Could you check a few things on this model? Use its own coordinates, in mm. A direction names the side the tool comes from. Give positions to 0.01 mm unless a question says otherwise; leave off trailing zeros. Loops run counter-clockwise (first coordinate to the right, second up) from the corner with the lowest first, then second, coordinate; pieces in that order, holes last. Notation, with made-up numbers: (-8, -27.5) -> (16, -27.5) arc R26 cw to (16, -8.5) -> close; hole circle Ø4 at (6.25, 21). An arc over 180 degrees is marked (long way). Write item = value, one per line. Start each with the question number.
1) I want a section at A-A (z = 8). List the corners of the cut face in (x, y) for me, and give its area (3 significant figures).
2) If we mould it in two halves opening along Y, with no side actions, what happens to faces 1 (the face through (17.3, -31.38, -17.42)), 2 (the face through (3, -33, -22)), 3 (the face through (14.026, 33.377, 10.944))? For each: +Y half, -Y half, draft (parallel to the pull), parting line (faces both ways), or undercut.
3) On a 3-axis mill with a long thin cutter (end or side, diameter ignored), from which of +Z, -Z, +X, -X, +Y, -Y can I reach the whole of each face in a straight line? I mean faces 4 (the face through (-17, 27, 15)), 5 (the face through (17.3, -31.38, 17.58)), 6 (the face through (-31.64, -11.92, 10.94)). Say none if no direction works.
4) I'm going to push flat-ended pins straight in: pin 1 Ø12 at (y, z) = (3, -14.5) entering from +X; pin 2 Ø2 at (y, z) = (28, -16.5) entering from +X; pin 3 Ø1.5 at (x, y) = (29.5, 11.5) entering from -Z. Where does each tip first touch, or does it pass through?
5) I need wall thicknesses on probe 1 along Z at (x, y) = (-17.5, -36.5); probe 2 along X at (y, z) = (0, 11); probe 3 along Y at (x, z) = (15, 10.5). Which ranges of each line are inside material? Lowest first, please. Write a range as from..to.
from build123d import *

# Parameters (mm, degrees)
EXTRUSION1_DEPTH              = 15
EXTRUSION1_DEPTH_BACK         = 15
SKETCH1_R                     = 37.5
SKETCH1_R_2                   = 31.15
CIRPATTERN1_COUNT             = 27
HOLE4_D                       = 2.5
HOLE4_DEPTH                   = 8
HOLE4_TIP                     = 1.25
EXTRUSION11_START             = 7
SKETCH5_R                     = 37.5
SKETCH5_R_2                   = 32.5
EXTRUSION11_DEPTH             = 7
SKETCH6_R                     = 37.5
SKETCH6_R_2                   = 32.5
EXTRUSION17_DEPTH             = 7
EXTRUSION18_REACH             = 59.415
EXTRUSION18_DIRECTION_2_REACH = 59.415
FILLET5_R                     = 20
HOLE6_D                       = 2.5
HOLE6_DEPTH                   = 8
HOLE6_TIP                     = 0.751075774


with BuildPart() as part:
    # Sketch1 → Extrusion1 (new, two sides: drawn at the far end of the back side and taken through both)
    with BuildSketch(Plane.XY.offset(-EXTRUSION1_DEPTH_BACK)):
        Circle(SKETCH1_R)
        Circle(SKETCH1_R_2, mode=Mode.SUBTRACT)
    extrusion1 = extrude(amount=EXTRUSION1_DEPTH + EXTRUSION1_DEPTH_BACK)


with BuildPart() as cirpattern1_1:
    # CirPattern1: pattern copy
    add(extrusion1.rotate(Axis((0, 0, 80.9), (0, 0, -1)), 1 * 360 / CIRPATTERN1_COUNT))


with BuildPart() as cirpattern1_2:
    # CirPattern1: pattern copy
    add(extrusion1.rotate(Axis((0, 0, 80.9), (0, 0, -1)), 2 * 360 / CIRPATTERN1_COUNT))


with BuildPart() as cirpattern1_3:
    # CirPattern1: pattern copy
    add(extrusion1.rotate(Axis((0, 0, 80.9), (0, 0, -1)), 3 * 360 / CIRPATTERN1_COUNT))


with BuildPart() as cirpattern1_4:
    # CirPattern1: pattern copy
    add(extrusion1.rotate(Axis((0, 0, 80.9), (0, 0, -1)), 4 * 360 / CIRPATTERN1_COUNT))


with BuildPart() as cirpattern1_5:
    # CirPattern1: pattern copy
    add(extrusion1.rotate(Axis((0, 0, 80.9), (0, 0, -1)), 5 * 360 / CIRPATTERN1_COUNT))


with BuildPart() as cirpattern1_6:
    # CirPattern1: pattern copy
    add(extrusion1.rotate(Axis((0, 0, 80.9), (0, 0, -1)), 6 * 360 / CIRPATTERN1_COUNT))


with BuildPart() as cirpattern1_7:
    # CirPattern1: pattern copy
    add(extrusion1.rotate(Axis((0, 0, 80.9), (0, 0, -1)), 7 * 360 / CIRPATTERN1_COUNT))


with BuildPart() as cirpattern1_8:
    # CirPattern1: pattern copy
    add(extrusion1.rotate(Axis((0, 0, 80.9), (0, 0, -1)), 8 * 360 / CIRPATTERN1_COUNT))


with BuildPart() as cirpattern1_9:
    # CirPattern1: pattern copy
    add(extrusion1.rotate(Axis((0, 0, 80.9), (0, 0, -1)), 9 * 360 / CIRPATTERN1_COUNT))


with BuildPart() as cirpattern1_10:
    # CirPattern1: pattern copy
    add(extrusion1.rotate(Axis((0, 0, 80.9), (0, 0, -1)), 10 * 360 / CIRPATTERN1_COUNT))


with BuildPart() as cirpattern1_11:
    # CirPattern1: pattern copy
    add(extrusion1.rotate(Axis((0, 0, 80.9), (0, 0, -1)), 11 * 360 / CIRPATTERN1_COUNT))


with BuildPart() as cirpattern1_12:
    # CirPattern1: pattern copy
    add(extrusion1.rotate(Axis((0, 0, 80.9), (0, 0, -1)), 12 * 360 / CIRPATTERN1_COUNT))


with BuildPart() as cirpattern1_13:
    # CirPattern1: pattern copy
    add(extrusion1.rotate(Axis((0, 0, 80.9), (0, 0, -1)), 13 * 360 / CIRPATTERN1_COUNT))


with BuildPart() as cirpattern1_14:
    # CirPattern1: pattern copy
    add(extrusion1.rotate(Axis((0, 0, 80.9), (0, 0, -1)), 14 * 360 / CIRPATTERN1_COUNT))


with BuildPart() as cirpattern1_15:
    # CirPattern1: pattern copy
    add(extrusion1.rotate(Axis((0, 0, 80.9), (0, 0, -1)), 15 * 360 / CIRPATTERN1_COUNT))


with BuildPart() as cirpattern1_16:
    # CirPattern1: pattern copy
    add(extrusion1.rotate(Axis((0, 0, 80.9), (0, 0, -1)), 16 * 360 / CIRPATTERN1_COUNT))


with BuildPart() as cirpattern1_17:
    # CirPattern1: pattern copy
    add(extrusion1.rotate(Axis((0, 0, 80.9), (0, 0, -1)), 17 * 360 / CIRPATTERN1_COUNT))


with BuildPart() as cirpattern1_18:
    # CirPattern1: pattern copy
    add(extrusion1.rotate(Axis((0, 0, 80.9), (0, 0, -1)), 18 * 360 / CIRPATTERN1_COUNT))


with BuildPart() as cirpattern1_19:
    # CirPattern1: pattern copy
    add(extrusion1.rotate(Axis((0, 0, 80.9), (0, 0, -1)), 19 * 360 / CIRPATTERN1_COUNT))


with BuildPart() as cirpattern1_20:
    # CirPattern1: pattern copy
    add(extrusion1.rotate(Axis((0, 0, 80.9), (0, 0, -1)), 20 * 360 / CIRPATTERN1_COUNT))


with BuildPart() as cirpattern1_21:
    # CirPattern1: pattern copy
    add(extrusion1.rotate(Axis((0, 0, 80.9), (0, 0, -1)), 21 * 360 / CIRPATTERN1_COUNT))


with BuildPart() as cirpattern1_22:
    # CirPattern1: pattern copy
    add(extrusion1.rotate(Axis((0, 0, 80.9), (0, 0, -1)), 22 * 360 / CIRPATTERN1_COUNT))


with BuildPart() as cirpattern1_23:
    # CirPattern1: pattern copy
    add(extrusion1.rotate(Axis((0, 0, 80.9), (0, 0, -1)), 23 * 360 / CIRPATTERN1_COUNT))


with BuildPart() as cirpattern1_24:
    # CirPattern1: pattern copy
    add(extrusion1.rotate(Axis((0, 0, 80.9), (0, 0, -1)), 24 * 360 / CIRPATTERN1_COUNT))


with BuildPart() as cirpattern1_25:
    # CirPattern1: pattern copy
    add(extrusion1.rotate(Axis((0, 0, 80.9), (0, 0, -1)), 25 * 360 / CIRPATTERN1_COUNT))


with BuildPart() as cirpattern1_26:
    # CirPattern1: pattern copy
    add(extrusion1.rotate(Axis((0, 0, 80.9), (0, 0, -1)), 26 * 360 / CIRPATTERN1_COUNT))


with BuildPart() as part_1:
    add(part.part)

    # CirPattern1 united with what the copies: union CirPattern1_1, CirPattern1_2, CirPattern1_3, CirPattern1_4, CirPattern1_5, CirPattern1_6, CirPattern1_7, CirPattern1_8, CirPattern1_9, CirPattern1_10, CirPattern1_11, CirPattern1_12, CirPattern1_13, CirPattern1_14, CirPattern1_15, CirPattern1_16, CirPattern1_17, CirPattern1_18, CirPattern1_19, CirPattern1_20, CirPattern1_21, CirPattern1_22, CirPattern1_23, CirPattern1_24, CirPattern1_25, CirPattern1_26
    add(cirpattern1_1.part)
    add(cirpattern1_2.part)
    add(cirpattern1_3.part)
    add(cirpattern1_4.part)
    add(cirpattern1_5.part)
    add(cirpattern1_6.part)
    add(cirpattern1_7.part)
    add(cirpattern1_8.part)
    add(cirpattern1_9.part)
    add(cirpattern1_10.part)
    add(cirpattern1_11.part)
    add(cirpattern1_12.part)
    add(cirpattern1_13.part)
    add(cirpattern1_14.part)
    add(cirpattern1_15.part)
    add(cirpattern1_16.part)
    add(cirpattern1_17.part)
    add(cirpattern1_18.part)
    add(cirpattern1_19.part)
    add(cirpattern1_20.part)
    add(cirpattern1_21.part)
    add(cirpattern1_22.part)
    add(cirpattern1_23.part)
    add(cirpattern1_24.part)
    add(cirpattern1_25.part)
    add(cirpattern1_26.part)

    # Hole4
    with Locations(Plane.XY.offset(15)):
        with Locations((35, 0), (13.862791811, 32.137563741), (-24.018457325, 25.458077455), (-32.889241728, -11.970705016), (-2.035069012, -34.940785539), (31.277142411, -15.707971307)):
            Hole(HOLE4_D / 2, depth=HOLE4_DEPTH)
            with Locations((0, 0, -(HOLE4_DEPTH + HOLE4_TIP / 2))):  # 90° drill point
                Cone(0, HOLE4_D / 2, HOLE4_TIP, mode=Mode.SUBTRACT)

    # Sketch5 → Extrusion11 (add)
    with BuildSketch(Plane(origin=(0, 0, -15), x_dir=(-1, 0, 0), z_dir=(0, 0, -1)).offset(EXTRUSION11_START)):
        with Locations(Location((0, 0, 0), (0, 0, 180))):
            Circle(SKETCH5_R)
        Circle(SKETCH5_R_2, mode=Mode.SUBTRACT)
    extrude(amount=-EXTRUSION11_DEPTH)

    # Sketch6 → Extrusion17 (add)
    with BuildSketch(Plane.XY.offset(15)):
        Circle(SKETCH6_R)
        with Locations(Location((0, 0, 0), (0, 0, 180))):
            Circle(SKETCH6_R_2, mode=Mode.SUBTRACT)
    extrude(amount=EXTRUSION17_DEPTH)

    # Extrusion18: up to this face of the body (flat: up to its plane)
    extrusion18_end = Plane(part_1.part.faces().sort_by_distance((-36.439339828, 0, 22))[0])
    # Sketch7 → Extrusion18 (add, up to the picked face)
    with BuildSketch(Plane.XY, mode=Mode.PRIVATE) as extrusion18_sk1:
        with BuildLine():
            Line((22.5, -40), (-22.5, -40))
            Line((-22.5, -40), (-22.5, -30))
            ThreePointArc((-22.5, -30), (0, -37.5), (22.5, -30))
            Line((22.5, -30), (22.5, -40))
        make_face()
    extrusion18_tool1 = split(extrude(extrusion18_sk1.sketch, amount=EXTRUSION18_REACH, mode=Mode.PRIVATE), bisect_by=extrusion18_end, keep=Keep.BOTH, mode=Mode.PRIVATE)
    add(extrusion18_tool1.solids().sort_by(Axis((22.039023, -35, 0), (0, 0, 1)))[0])

    # Extrusion18 direction 2: up to this face of the body (flat: up to its plane)
    extrusion18_direction_2_end = Plane(part_1.part.faces().sort_by_distance((-36.439339828, 0, -22))[0])
    # Sketch7 → Extrusion18 direction 2 (add, up to the picked face)
    with BuildSketch(Plane.XY, mode=Mode.PRIVATE) as extrusion18_direction_2_sk1:
        with BuildLine():
            Line((22.5, -40), (-22.5, -40))
            Line((-22.5, -40), (-22.5, -30))
            ThreePointArc((-22.5, -30), (0, -37.5), (22.5, -30))
            Line((22.5, -30), (22.5, -40))
        make_face()
    extrusion18_direction_2_tool1 = split(extrude(extrusion18_direction_2_sk1.sketch, amount=-EXTRUSION18_DIRECTION_2_REACH, mode=Mode.PRIVATE), bisect_by=extrusion18_direction_2_end, keep=Keep.BOTH, mode=Mode.PRIVATE)
    add(extrusion18_direction_2_tool1.solids().sort_by(Axis((22.039023, -35, 0), (0, 0, -1)))[0])

    # Fillet5
    fillet5_edges = [part_1.edges().sort_by_distance(p)[0] for p in [
        (22.5, -30, 0),
        (-22.5, -30, 0),
    ]]
    fillet(fillet5_edges, radius=FILLET5_R)

    # Sketch8 → Revolution1 (revolve, cut)
    with BuildSketch(Plane.YZ, mode=Mode.PRIVATE) as revolution1_sk:
        Polygon((31.493036454, 15), (30.493036454, 15), (30.493036454, 14), align=None)
    revolution1 = revolve(revolution1_sk.sketch.rotate(Axis((0, 0, 0), (0, 0, 1)), 270), axis=Axis((0, 0, 0), (0, 0, 1)), mode=Mode.SUBTRACT)

    # Mirror1: Revolution1 across plane
    add(revolution1.mirror(Plane.XY), mode=Mode.SUBTRACT)

    # Hole6
    with Locations(Plane(origin=(0, -40, 0), x_dir=(-1, 0, 0), z_dir=(0, -1, 0))):
        with Locations((-17.5, -17.5), (-17.5, 17.5), (17.5, -17.5), (17.5, 17.5)):
            Hole(HOLE6_D / 2, depth=HOLE6_DEPTH)
            with Locations((0, 0, -(HOLE6_DEPTH + HOLE6_TIP / 2))):  # 118° drill point
                Cone(0, HOLE6_D / 2, HOLE6_TIP, mode=Mode.SUBTRACT)


solid = part_1.part
Answer list:
q1.outline = (-27.72, -25.26) arc R20 cw to (-22.5, -38.73) -> (-22.5, -40) -> (22.5, -40) -> (22.5, -38.73) arc R20 cw to (27.72, -25.26) arc R37.5 ccw (long way) to start; hole circle Ø2.5 at (-32.89, -11.97); hole circle Ø62.3 at (0, 0); hole circle Ø2.5 at (-24.02, 25.46); hole circle Ø2.5 at (-2.04, -34.94); hole circle Ø2.5 at (13.86, 32.14); hole circle Ø2.5 at (31.28, -15.71); hole circle Ø2.5 at (35, 0)
q1.area = 1,580 mm^2
q2.face_1 = -Y half
q2.face_2 = draft
q2.face_3 = undercut
q3.face_4 = +Z
q3.face_5 = -Y
q3.face_6 = none
q4.pin_1 = 37.5
q4.pin_2 = 26.02
q4.pin_3 = -15
q5.probe_1 = -22..-18.75, -16.25..16.25, 18.75..22
q5.probe_2 = -37.5..-31.15, 31.15..33.75, 36.25..37.5
q5.probe_3 = -40..-27.3, 27.3..31.62, 32.66..34.37
